Input: dimensioned drawing with shaded views. Units: mm. Origin: part minimum x, y, z. Give positions to 0.01 mm unless a question says otherwise; leave off trailing zeros. Loops run counter-clockwise (first coordinate to the right, second up) from the corner with the lowest first, then second, coordinate; pieces in that order, holes last. Notation, with made-up numbers: (72.5, -19.5) -> (100.5, -19.5) arc R11 ccw to (100.5, -3.5) -> close; hole circle Ø1 at (40.25, -28). An arc over 180 degrees is marked (long way). Answer as a JSON object with one key per item and string values.
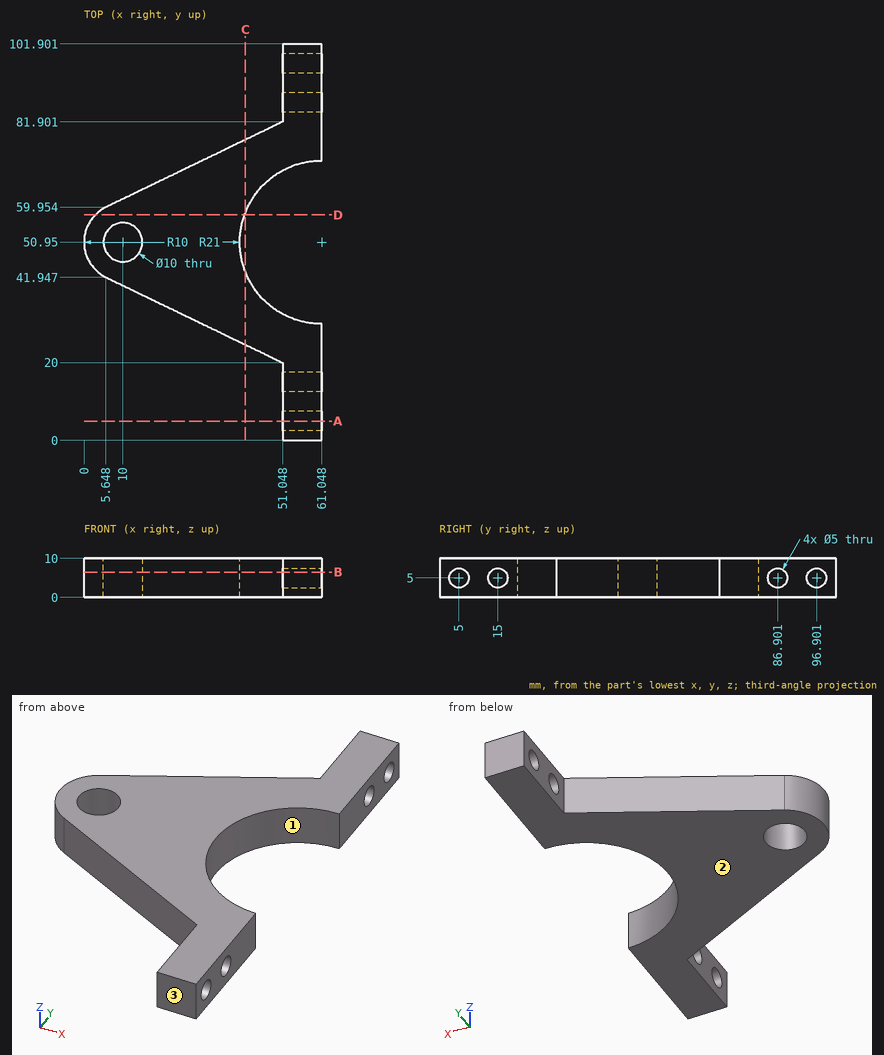
Q1. Ray query, line 1 along Z through (x, y) = (58.5, 5); line 2 along Y through (x, z) = (58, 5); line 3 along Y through (x, z) = (54, 5). Return the intervals inside material, ascending.
Evaluation:
{"line 1": "z = 0 to 2.5, 7.5 to 10", "line 2": "y = 0 to 2.5, 7.5 to 12.5, 17.5 to 30.17, 71.73 to 84.4, 89.4 to 94.4, 99.4 to 101.9", "line 3": "y = 0 to 2.5, 7.5 to 12.5, 17.5 to 31.17, 70.73 to 84.4, 89.4 to 94.4, 99.4 to 101.9"}
Q2. Section A-A, the plane y = 5. Return the cut outline in (x, z).
Evaluation:
{"outline": "(51.05, 0) -> (61.05, 0) -> (61.05, 2.5) -> (51.05, 2.5) -> close; (51.05, 7.5) -> (61.05, 7.5) -> (61.05, 10) -> (51.05, 10) -> close"}
Q3. Pin query (flat end, axial travel): pin 1 (5 mm diameter, centred on y = 52.5, z = 4, fed in from +X); pin 2 (4 mm diameter, centred on x = 47, z = 7, fed in from -Y); pin 3 (4.5 mm diameter, centred on y = 15, z = 5, fed in from -X); pin 4 (2 mm diameter, centred on y = 57, z = 1.5, fed in from -X). Return the tip coordinate at first contact, or that it passes through.
Evaluation:
{"pin 1": "stops at x = 40.44", "pin 2": "stops at y = 20.99", "pin 3": "passes through", "pin 4": "stops at x = 1.37"}
Q4. Section B-B, the plane z = 6.5. Return the cut outline in (x, y), then the cut area to 3 significant figures.
Evaluation:
{"outline": "(5.65, 41.95) -> (51.05, 20) -> (51.05, 17) -> (61.05, 17) -> (61.05, 29.95) arc R21 cw to (61.05, 71.95) -> (61.05, 84.9) -> (51.05, 84.9) -> (51.05, 81.9) -> (5.65, 59.95) arc R10 ccw to start; (51.05, 0) -> (61.05, 0) -> (61.05, 3) -> (51.05, 3) -> close; (51.05, 7) -> (61.05, 7) -> (61.05, 13) -> (51.05, 13) -> close; (51.05, 88.9) -> (61.05, 88.9) -> (61.05, 94.9) -> (51.05, 94.9) -> close; (51.05, 98.9) -> (61.05, 98.9) -> (61.05, 101.9) -> (51.05, 101.9) -> close; hole circle Ø10 at (10, 50.95)", "area": "1,970 mm2"}
Q5. Section D-D, the plane y = 58. Return the cut outline in (x, z).
Evaluation:
{"outline": "(2.91, 0) -> (41.27, 0) -> (41.27, 10) -> (2.91, 10) -> close"}
Q6. Draft query along Y for the marked faces 1, 2 and 3. Return one class per face: +Y half, -Y half, draft (parallel to the pull), parting line (faces both ways), or undercut.
Evaluation:
{"face 1": "undercut", "face 2": "draft", "face 3": "-Y half"}
Q7. Section C-C, the plane x = 41.5. Return the cut outline in (y, z) (1 decimal).
Evaluation:
{"outline": "(24.6, 0) -> (43.3, 0) -> (43.3, 10) -> (24.6, 10) -> close; (58.6, 0) -> (77.3, 0) -> (77.3, 10) -> (58.6, 10) -> close"}
